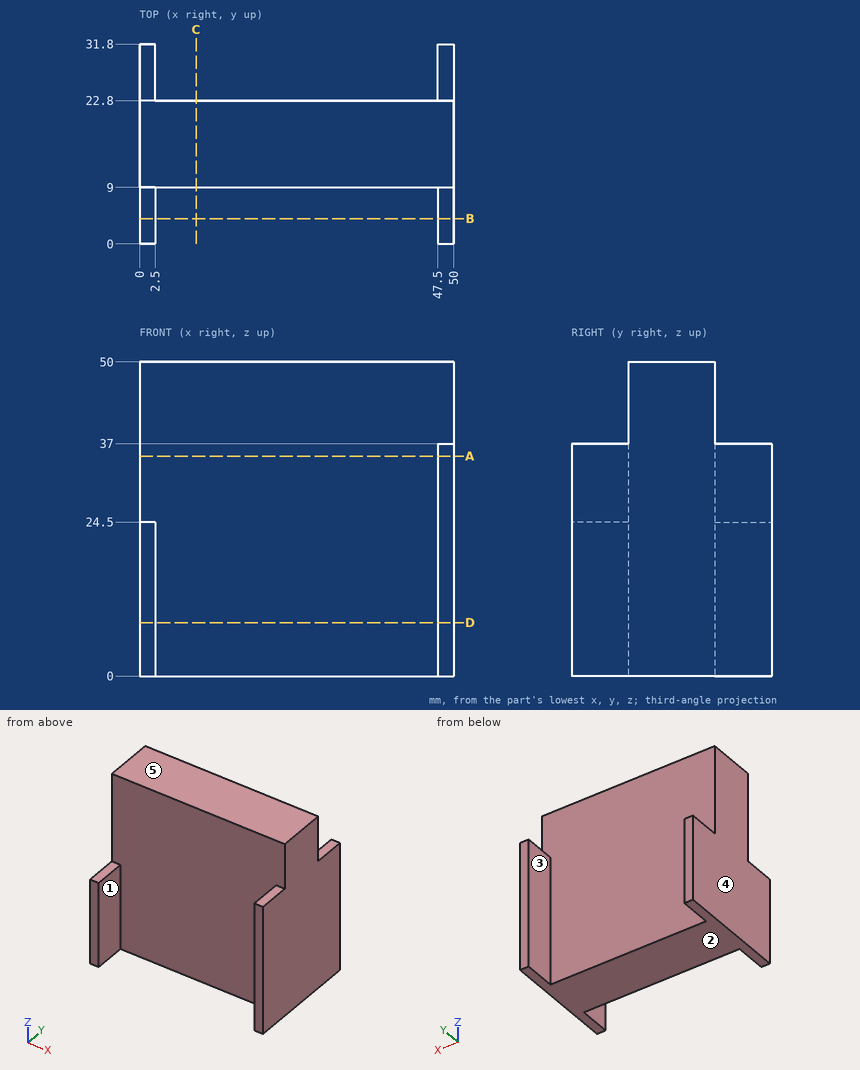
Can you work these out from the drawing? Everything is in mm from the part's minimum corner. A direction names the side the tool comes from. Round coordinates to 2 decimals unless told otherwise and drop trailing zeros. Loops run counter-clockwise (first coordinate to the right, second up) from the corner with the lowest first, then second, coordinate; pieces in that order, holes last. Notation, with made-up numbers: M 54,82.25 L 78,82.25 A28 ccw 78,118.25 Z; hole C 73.25,1.5 d9. An arc over 180 degrees is marked long. Write item = value, one per line.
1. I want a section at D-D, the plane z = 8.5. Write out the boundary of the cut face in (x, y).
Results below:
outline = M 0,0 L 2.5,0 L 2.5,9 L 47.5,9 L 47.5,0 L 50,0 L 50,31.8 L 47.5,31.8 L 47.5,22.8 L 2.5,22.8 L 2.5,31.8 L 0,31.8 Z
2. I want a section at A-A, the plane z = 35. Write out the boundary of the cut face in (x, y).
Results below:
outline = M 0,9 L 47.5,9 L 47.5,0 L 50,0 L 50,31.8 L 47.5,31.8 L 47.5,22.8 L 0,22.8 Z
3. I want a section at B-B, the plane y = 4. Write out the boundary of the cut face in (x, z).
Results below:
outline = M 0,0 L 2.5,0 L 2.5,24.5 L 0,24.5 Z; M 47.5,0 L 50,0 L 50,37 L 47.5,37 Z
4. I want a section at C-C, the plane x = 9. Write out the boundary of the cut face in (y, z), and give its area (3 significant figures).
Results below:
outline = M 9,0 L 22.8,0 L 22.8,50 L 9,50 Z
area = 690 mm²
5. Thinking about a two-plate mould opening in X: for the marked faces 3, 4 and 5, which applies, +X half, -X half, draft (parallel to the pull), parting line (faces both ways), or undercut?
Results below:
face_3 = undercut
face_4 = -X half
face_5 = draft
6. I need wall thicknesses on probe 1 along X at (y, z) = (26, 24); probe 2 along Y at (x, z) = (29.5, 46.5); probe 3 along X at (y, z) = (27.5, 29). Which ranges of each line are inside material? Lowest first, please.
Results below:
probe_1 = 0 to 2.5, 47.5 to 50
probe_2 = 9 to 22.8
probe_3 = 47.5 to 50
7. Which directions (+Z, -Z, +X, -X, +Y, -Y) give clear straight access to the entire face, cutting with the end or side of a thin tool? Please do the marked faces 1 and 2.
Results below:
face_1 = +Z, -Z, -Y
face_2 = -Z, +X, -X, +Y, -Y
8. Will these pins go through, and if not, where does the flat tip stop? P1, Ø2, axis at x = 2, y = 5, coming from the +Z side; P2, Ø3, axis at x = 48.5, y = 5, coming from the +Z side; P3, Ø2, axis at x = 41, z = 26, coming from the +Y side.
Results below:
P1 = 24.5
P2 = 37
P3 = 22.8
